Geometry check sheet. Reference: the model listing, model coordinates, mm. Round coordinates to 2 decimals unless told otherwise and drop trailing zeros. Write each loop counter-clockwise with the first axis right and the second up, starting at its lowest first coordinate (ties: lowest second). Pieces come first, ordered by that corner, then holes.
Item 1: Cross-section at A-A (y = -4.5). Enter the section's corners in (x, z).
Item 2: Scan lines: probe 1 along Z at (x, y) = (965, 6.5); probe 2 along Y at (x, z) = (933, 23). Record each from-to range of solid material in increasing order.
Item 3: Cross-section at B-B (x = 361). Enter the section's corners in (y, z) (3 decimals), then the cut area to 3 significant figures.
Autodesk Inventor part; units mm, degrees
ref_plane "YZ Plane" through (0, 0, 0) normal (1, 0, 0) x (0, 1, 0)
ref_plane "XZ Plane" through (0, 0, 0) normal (0, 1, 0) x (-1, 0, 0)
ref_plane "XY Plane" through (0, 0, 0) normal (0, 0, 1) x (1, 0, 0)
sketch "Sketch1" plane through (0, 0, 0) normal (1, 0, 0) x (0, 1, 0)
  line L0 (25.4, 25.4) -> (-25.4, 25.4)
  line L1 (-25.4, 25.4) -> (-25.4, -25.4)
  line L2 (-25.4, -25.4) -> (25.4, -25.4)
  line L3 (25.4, -25.4) -> (25.4, 25.4)
  line L4 (23.2918, 23.2918) -> (-23.2918, 23.2918)
  line L5 (-23.2918, 23.2918) -> (-23.2918, -23.2918)
  line L6 (-23.2918, -23.2918) -> (23.2918, -23.2918)
  line L7 (23.2918, -23.2918) -> (23.2918, 23.2918)
  point P0 (0, 0)
  point P1 (0, -25.4)
  point P2 (25.4, 0)
  dimension "d0" = 50.8
  dimension "d1" = 50.8
  dimension "d2" = 2.1082
extrude "Extrusion1" add sketch "Sketch1" along normal blind 1016
fillet "Fillet1" radius 3.175 4 edges at (508, 25.4, 25.4) (508, -25.4, 25.4) (508, 25.4, -25.4) (508, -25.4, -25.4)
properties part number "48_Inch_square" material "Steel"
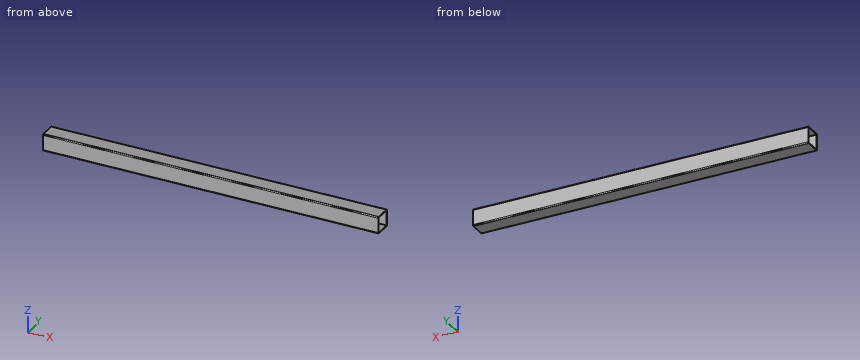
Resolved:
1. outline: (0, -25.4) - (1016, -25.4) - (1016, -23.29) - (0, -23.29) - close; (0, 23.29) - (1016, 23.29) - (1016, 25.4) - (0, 25.4) - close
2. probe 1: z = -25.4 to -23.29, 23.29 to 25.4
2. probe 2: y = -25.3 to -23.29, 23.29 to 25.3
3. outline: (-25.4, -22.225) arc R3.175 ccw to (-22.225, -25.4) - (22.225, -25.4) arc R3.175 ccw to (25.4, -22.225) - (25.4, 22.225) arc R3.175 ccw to (22.225, 25.4) - (-22.225, 25.4) arc R3.175 ccw to (-25.4, 22.225) - close; hole (-23.292, -23.292) - (23.292, -23.292) - (23.292, 23.292) - (-23.292, 23.292) - close
3. area: 402 mm2
